```python
from build123d import *

# Parameters (mm, degrees)
SKETCH1_R           = 4
BOSS_EXTRUDE1_DEPTH = 73
SKETCH2_W           = 0.5
SKETCH2_H           = 1


with BuildPart() as part:
    # Sketch1 → Boss-Extrude1 (new body)
    with BuildSketch(Plane(origin=(0, 0, 0), x_dir=(1, 0, 0), z_dir=(0, 1, 0))):
        Circle(SKETCH1_R)
    extrude(amount=BOSS_EXTRUDE1_DEPTH)

    # Sketch2 → Cut-Revolve1 (revolve, cut)
    with BuildSketch(Plane.XY):
        with Locations((-3.75, 57.5)):
            Rectangle(SKETCH2_W, SKETCH2_H)
        with Locations((-3.75, 2.5)):
            Rectangle(SKETCH2_W, SKETCH2_H)
    revolve(axis=Axis((0, 73, 0), (0, -1, 0)), mode=Mode.SUBTRACT)


solid = part.part
```
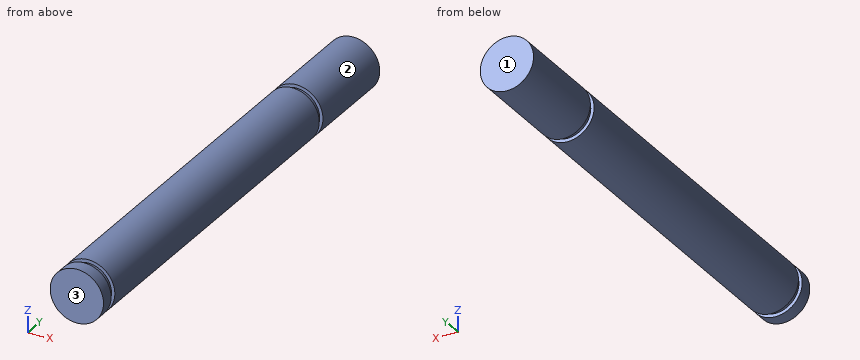
Could you check a few things on this model? Use its own coordinates, in mm. Face numbers are marked on the shaded views. Coordinates: 2 decimals unless noted, no trailing zeros. Write each loop counter-clockwise with the first axis right and the second up, starting at its lowest first coordinate (ties: lowest second). Pieces come first, ordered by that corner, then holes. Notation, with made-up numbers: (-15, 31) - (-9, 31) arc R8 cw to (-9, 42) - close; hole circle Ø1 at (6.25, -33). An arc over 180 degrees is marked (long way). Use a Markdown table: item, result.
Q1. I'm going to push flat-ended pins straight in: pin 1 Ø3 at (y, z) = (31, -2) entering from +X; pin 2 Ø1 at (x, y) = (-1, 39) entering from +Z; pin 3 Ø3 at (y, z) = (35, 2.5) entering from +X. Where does each tip first touch, or does it pass through?
Geometry check:
| item | result |
|---|---|
| pin 1 | stops at x = 3.97 |
| pin 2 | stops at z = 3.97 |
| pin 3 | stops at x = 3.87 |
Q2. Thinking about a two-plate mould opening in Y: for the marked faces 1, 2 and 3, which applies, +Y half, -Y half, draft (parallel to the pull), parting line (faces both ways), or undercut?
Geometry check:
| item | result |
|---|---|
| face 1 | +Y half |
| face 2 | draft |
| face 3 | -Y half |
Q3. Please list where these lines run through material, in increasing order: L1, parallel to Y at x = 2.5, z = 3; L2, parallel to X at y = 53.5, z = 0.25.
Geometry check:
| item | result |
|---|---|
| L1 | y = 0 to 2, 3 to 57, 58 to 73 |
| L2 | x = -3.99 to 3.99 |
Q4. Imagine slicing it at B-B (x = -1.5). List the corners of the cut face in (y, z) for me, and give its area (3 significant figures).
Geometry check:
| item | result |
|---|---|
| outline | (0, -3.71) - (2, -3.71) - (2, -3.16) - (3, -3.16) - (3, -3.71) - (57, -3.71) - (57, -3.16) - (58, -3.16) - (58, -3.71) - (73, -3.71) - (73, 3.71) - (58, 3.71) - (58, 3.16) - (57, 3.16) - (57, 3.71) - (3, 3.71) - (3, 3.16) - (2, 3.16) - (2, 3.71) - (0, 3.71) - close |
| area | 539 mm2 |
Q5. Imagine slicing it at A-A (z = 2). List the corners of the cut face in (x, y) for me.
Geometry check:
| item | result |
|---|---|
| outline | (-3.46, 0) - (3.46, 0) - (3.46, 2) - (2.87, 2) - (2.87, 3) - (3.46, 3) - (3.46, 57) - (2.87, 57) - (2.87, 58) - (3.46, 58) - (3.46, 73) - (-3.46, 73) - (-3.46, 58) - (-2.87, 58) - (-2.87, 57) - (-3.46, 57) - (-3.46, 3) - (-2.87, 3) - (-2.87, 2) - (-3.46, 2) - close |
